Can you work these out from the model? Positions are in its coordinate system, mm. A direction names the side the tool comes from. Round coordinates to 2 decimals unless told otherwise and drop trailing zeros. Loops run counter-clockwise (first coordinate to the right, second up) from the corner with the lowest first, then second, coordinate; pieces in that order, holes last.
from build123d import *

# Parameters (mm, degrees)
F0_W      = 114.3
F0_H      = 114.3
F1_DEPTH  = 12.7
F2_R      = 50.8635
F3_DEPTH  = 6.477
F4_R      = 44.5135
F5_DEPTH  = 6.224
F6_R      = 9.525
F8_D      = 5.1054
F9_R      = 110.5427806282
F9_R_2    = 63.5
F10_DEPTH = 25.4
F12_D     = 5.1054


with BuildPart() as f1:
    # F0 (on Front) → F1 (new body)
    with BuildSketch(Plane.XZ):
        Rectangle(F0_W, F0_H)
    extrude(amount=-F1_DEPTH)

    # F2 (on face) → F3 (cut)
    with BuildSketch(Plane(origin=(0, 12.7, 0), x_dir=(-1, 0, 0), z_dir=(0, 1, 0))):
        Circle(F2_R)
    extrude(amount=-F3_DEPTH, mode=Mode.SUBTRACT)

    # F4 (on face) → F5 (cut, through all)
    with BuildSketch(Plane(origin=(0, 6.223, 0), x_dir=(-1, 0, 0), z_dir=(0, 1, 0))):
        Circle(F4_R)
    extrude(amount=-F5_DEPTH, mode=Mode.SUBTRACT)

    # F6
    f6_edges = [f1.edges().sort_by_distance(p)[0] for p in [
        (57.15, 6.35, 57.15),
        (-57.15, 6.35, 57.15),
        (57.15, 6.35, -57.15),
        (-57.15, 6.35, -57.15),
    ]]
    fillet(f6_edges, radius=F6_R)

    # F8 (through all)
    with Locations(Plane(origin=(0, 12.7, 0), x_dir=(-1, 0, 0), z_dir=(0, 1, 0))):
        with Locations((-47.625, 47.625), (47.625, -47.625), (47.625, 47.625), (-47.625, -47.625)):
            Hole(F8_D / 2)

    # F9 (on Front) → F10 (cut)
    with BuildSketch(Plane.XZ):
        Circle(F9_R)
        Circle(F9_R_2, mode=Mode.SUBTRACT)
    extrude(amount=-F10_DEPTH, mode=Mode.SUBTRACT)

    # F12 (through all)
    with Locations(Plane(origin=(0, 12.7, 0), x_dir=(-1, 0, 0), z_dir=(0, 1, 0))):
        with Locations((40.4111525448, 40.4111525448), (-40.4111525448, 40.4111525448), (-40.4111525448, -40.4111525448), (40.4111525448, -40.4111525448)):
            Hole(F12_D / 2)


solid = f1.part
(1) If we section it at A-A, the plane z = 0: List the corners of the cut face in (x, y) for me, then the cut area to 3 significant figures.
Worked answers:
outline: (-57.15, 0) - (-44.51, 0) - (-44.51, 6.22) - (-50.86, 6.22) - (-50.86, 12.7) - (-57.15, 12.7) - close; (44.51, 0) - (57.15, 0) - (57.15, 12.7) - (50.86, 12.7) - (50.86, 6.22) - (44.51, 6.22) - close
area: 239 mm2
(2) If we mould it in two halves opening along X, with no side actions, what happens to faces 3 (the cylindrical face through (45.1, 6.3, 44.7)), 4 (the flat face through (0, 6.223, -45)), 5 (the flat face through (-57.15, 6, 0)), 6 (the cylindrical face through (42.846, 6.261, -39.644))? For each: released by +X, released by -X, zero draft, split by the parting line, or undercut.
Worked answers:
face 3: released by +X
face 4: undercut
face 5: released by -X
face 6: undercut
(3) If we section it at B-B, the plane x = -9: List the corners of the cut face in (y, z) for me, then the cut area to 3 significant figures.
Worked answers:
outline: (0, -57.15) - (12.7, -57.15) - (12.7, -50.06) - (6.22, -50.06) - (6.22, -43.59) - (0, -43.59) - close; (0, 43.59) - (6.22, 43.59) - (6.22, 50.06) - (12.7, 50.06) - (12.7, 57.15) - (0, 57.15) - close
area: 261 mm2
(4) If we section it at C-C, the plane y = 3: List the corners of the cut face in (x, z) for me, then the cut area to 3 significant figures.
Worked answers:
outline: (-57.15, -27.68) arc R63.5 ccw to (-27.68, -57.15) - (27.68, -57.15) arc R63.5 ccw to (57.15, -27.68) - (57.15, 27.68) arc R63.5 ccw to (27.68, 57.15) - (-27.68, 57.15) arc R63.5 ccw to (-57.15, 27.68) - close; hole circle Ø89.03 at (0, 0); hole circle Ø5.11 at (-40.41, -40.41); hole circle Ø5.11 at (-40.41, 40.41); hole circle Ø5.11 at (40.41, -40.41); hole circle Ø5.11 at (40.41, 40.41)
area: 5,410 mm2
(5) Will these pins go through, and if not, where does the flat tip stop? P1, Ø6.5, axis at x = 40.41, z = -40.41, coming from the +Y side; P2, Ø5, axis at y = 3, z = -40, coming from the +X side; P3, Ø5, axis at x = 1.5, z = 45, coming from the +Y side.
Worked answers:
P1: stops at y = 12.7
P2: stops at x = 51.24
P3: stops at y = 6.22
(6) If we section it at D-D, the plane x = -41: List the corners of the cut face in (y, z) for me (3 decimals).
Worked answers:
outline: (0, -48.49) - (12.7, -48.49) - (12.7, -42.895) - (0, -42.895) - close; (0, -37.927) - (12.7, -37.927) - (12.7, -30.101) - (6.223, -30.101) - (6.223, -17.334) - (0, -17.334) - close; (0, 17.334) - (6.223, 17.334) - (6.223, 30.101) - (12.7, 30.101) - (12.7, 37.927) - (0, 37.927) - close; (0, 42.895) - (12.7, 42.895) - (12.7, 48.49) - (0, 48.49) - close
(7) For faces 1 (the cylindrical face through (41.783, 6.261, 42.564)), 2 (the cylindrical face through (-48.515, 9.507, 15.278)), which set-ups out of +Z, -Z, +X, -X, +Y, -Y let a thin tool reach every point of the face, with its end or its side?
Worked answers:
face 1: +Y, -Y
face 2: +Y
(8) If I drill on line 1 (Z direction, x = -1, y = 5.5); line 2 (X direction, y = 6.5, z = -42.5); line 3 (X direction, y = 4.25, z = -36), over which ranges is the centre line in solid material (lowest first)?
Worked answers:
line 1: z = -57.15 to -44.5, 44.5 to 57.15
line 2: x = -47.18 to -41.88, -38.94 to -27.94, 27.94 to 38.94, 41.88 to 47.18
line 3: x = -52.31 to -26.18, 26.18 to 52.31
